from build123d import *
from build123d.topology import SkipClean

# Parameters (mm, degrees)
BOSS_EXTRUDE1_DEPTH      = 20
CUT_EXTRUDE1_DEPTH       = 60.487961127
BOSS_EXTRUDE2_DEPTH      = 4
CHAMFER1_SIZE            = 4
BOSS_EXTRUDE3_DEPTH      = 30
BOSS_EXTRUDE3_DEPTH_BACK = 80
CUT_EXTRUDE2_DEPTH       = 163.896367878
SHELL1_START             = -17.663350197
SHELL1_DEPTH             = 97.938189841
SHELL1_START_2           = -19.725064534
SHELL1_2_OUTLINE_W       = 18
SHELL1_2_OUTLINE_H       = 46
SHELL1_2_DEPTH           = 3.170813997
SHELL1_START_3           = 4.138253986
SHELL1_3_DEPTH           = 15.861746014
SHELL1_START_4           = -11.021607192
SHELL1_4_DEPTH           = 5.325277307
SHELL1_START_5           = -5.696329885
SHELL1_5_DEPTH           = 2


with BuildPart() as part:
    # Sketch1 → Boss-Extrude1 (new body)
    with BuildSketch(Plane(origin=(0, 0, 0), x_dir=(1, 0, 0), z_dir=(0, 1, 0))):
        with BuildLine():
            Line((25.274839644, -23.491941756), (25.274839644, 16.508058244))
            Line((25.274839644, 16.508058244), (-18.05582698, 16.508058244))
            ThreePointArc((-18.05582698, 16.508058244), (-21.573303396, -3.353843819), (-20.422301498, -23.491941756))
            ThreePointArc((-20.422301498, -23.491941756), (-19.386839701, -28.526912443), (-18.05582698, -33.491941756))
            Line((-18.05582698, -33.491941756), (25.274839644, -33.491941756))
            Line((25.274839644, -33.491941756), (25.274839644, -23.491941756))
        make_face()
    extrude(amount=BOSS_EXTRUDE1_DEPTH)

    # Sketch2 → Cut-Extrude1 (cut, through all)
    with BuildSketch(Plane.XY.offset(33.491941756)):
        Polygon((-18.05582698, 10), (-18.05582698, 0), (-8.05582698, 0), align=None)
        Polygon((-8.05582698, 0), (-18.05582698, 0), (-18.05582698, 10), (-26.022793605, 17.966966625), (-26.022793605, -4.913514026), (-8.05582698, -4.913514026), align=None)
    extrude(amount=-CUT_EXTRUDE1_DEPTH, mode=Mode.SUBTRACT)

    # Sketch3 → Boss-Extrude2 (add)
    with BuildSketch(Plane(origin=(0, 20, 0), x_dir=(1, 0, 0), z_dir=(0, 1, 0))):
        with BuildLine():
            Line((-20.591335302, 5.508058244), (-18.56429203, 5.508058244))
            ThreePointArc((-18.56429203, 5.508058244), (-19.725160356, -8.491941756), (-18.56429203, -22.491941756))
            Line((-18.56429203, -22.491941756), (-20.591335302, -22.491941756))
            ThreePointArc((-20.591335302, -22.491941756), (-21.725160356, -8.491941756), (-20.591335302, 5.508058244))
        make_face()
    extrude(amount=BOSS_EXTRUDE2_DEPTH)

    # Chamfer1
    chamfer1_edges = [part.edges().sort_by_distance(p)[0] for p in [
        (-19.577813666, 24, -5.508058244),
        (-19.577813666, 24, 22.491941756),
    ]]
    chamfer(chamfer1_edges, length=CHAMFER1_SIZE - 0.0001)  # a hair under: the kernel refuses the full size

    # Sketch4 → Boss-Extrude3 (add, two sides: drawn at the far end of the back side and taken through both)
    with BuildSketch(Plane.XY.offset(33.491941756).offset(-BOSS_EXTRUDE3_DEPTH_BACK)):
        Polygon((65.274839644, 110), (57.510268291, 81.022225211), (25.274839644, 20), (25.274839644, 0), (80.274839644, 0), (80.274839644, 110), align=None)
    extrude(amount=BOSS_EXTRUDE3_DEPTH + BOSS_EXTRUDE3_DEPTH_BACK)

    # Sketch5 → Cut-Extrude2 (cut, through all)
    with BuildSketch(Plane(origin=(80.274839644, 0, 0), x_dir=(0, 0, -1), z_dir=(1, 0, 0))):
        Polygon((-63.491941756, 0), (-33.491941756, 0), (-33.491941756, 30), (-63.491941756, 81.022225211), align=None)
    cut_extrude2 = extrude(amount=-CUT_EXTRUDE2_DEPTH, mode=Mode.SUBTRACT)

    # Mirror1: Cut-Extrude2 across plane
    add(cut_extrude2.mirror(Plane.XY.offset(8.491941756)), mode=Mode.SUBTRACT)

    # Shell1: read off the stored shape, not the designer's step
    # Shell1 outline → Shell1 (cut)
    with BuildSketch(Plane.YZ.offset(SHELL1_START)):
        Polygon((2, 31.491941756), (2, -14.508058244), (30.544412087, -14.508058244), (81.566637298, -44.508058244), (110, -44.508058244), (110, 61.491941756), (81.566637298, 61.491941756), (30.544412087, 31.491941756), align=None)
    extrude(amount=SHELL1_DEPTH, mode=Mode.SUBTRACT)

    # Shell1 2 outline → Shell1 2 (cut)
    with BuildSketch(Plane.YZ.offset(SHELL1_START_2)):
        with Locations((11, 8.491941756)):
            Rectangle(SHELL1_2_OUTLINE_W, SHELL1_2_OUTLINE_H)
    extrude(amount=SHELL1_2_DEPTH, mode=Mode.SUBTRACT)

    # Shell1 3 outline → Shell1 3 (add)
    with SkipClean():  # the faces are left unmerged after this step: merging them gives an invalid solid
        with BuildSketch(Plane(origin=(0, 0, 0), x_dir=(1, 0, 0), z_dir=(0, 1, 0)).offset(SHELL1_START_3)):
            with BuildLine():
                ThreePointArc((-19.725064534, -27.039617882), (-19.20680208, -29.272995907), (-18.62986821, -31.491941756))
                Line((-18.62986821, -31.491941756), (-16.554250537, -31.491941756))
                ThreePointArc((-16.554250537, -31.491941756), (-18.92870145, -20.100717198), (-19.725160356, -8.491941756))
                Line((-19.725160356, -8.491941756), (-19.725064534, -27.039617882))
            make_face()
            with BuildLine():
                ThreePointArc((-18.62986821, 14.508058244), (-19.20680208, 12.289112394), (-19.725064535, 10.055734369))
                Line((-19.725064535, 10.055734369), (-19.725160356, -8.491941756))
                ThreePointArc((-19.725160356, -8.491941756), (-18.92870145, 3.116833686), (-16.554250537, 14.508058244))
                Line((-16.554250537, 14.508058244), (-18.62986821, 14.508058244))
            make_face()
        extrude(amount=SHELL1_3_DEPTH)

    # Shell1 4 outline → Shell1 4 (cut)
    with SkipClean():  # the faces are left unmerged after this step: merging them gives an invalid solid
        with BuildSketch(Plane(origin=(0, 0, 0), x_dir=(0.7071067811865509, -0.707106781186544, 0), z_dir=(0.707106781186544, 0.707106781186551, 0)).offset(SHELL1_START_4)):
            with BuildLine():
                Line((-5.696329885, 16.508058244), (-19.838465509, 16.508058244))
                add(Edge.make_bspline(
                    [(-19.838465509, 16.508058244), (-30.445406654, -8.491941756), (-19.838465509, -33.491941756)],
                    knots=[2.850127051, 2.850127051, 2.850127051, 3.433058256, 3.433058256, 3.433058256], degree=2, weights=[1, 0.957823754, 1]))
                Line((-19.838465509, -33.491941756), (-5.696329885, -33.491941756))
                Line((-5.696329885, -33.491941756), (-5.696329885, 16.508058244))
            make_face()
        extrude(amount=SHELL1_4_DEPTH, mode=Mode.SUBTRACT)

    # Shell1 5 outline → Shell1 5 (add)
    with SkipClean():  # the faces are left unmerged after this step: merging them gives an invalid solid
        with BuildSketch(Plane(origin=(0, 0, 0), x_dir=(0.7071067811865509, -0.707106781186544, 0), z_dir=(0.707106781186544, 0.707106781186551, 0)).offset(SHELL1_START_5)):
            with BuildLine():
                Line((-6.52475701, -31.491941756), (-6.52475701, 14.508058244))
                Line((-6.52475701, 14.508058244), (-19.71491574, 14.508058244))
                add(Edge.make_bspline(
                    [(-19.71491574, 14.508058244), (-28.857373182, -8.491941756), (-19.71491574, -31.491941756)],
                    knots=[2.867588645, 2.867588645, 2.867588645, 3.415596662, 3.415596662, 3.415596662], degree=2, weights=[1, 0.962695179, 1]))
                Line((-19.71491574, -31.491941756), (-6.52475701, -31.491941756))
            make_face()
        extrude(amount=SHELL1_5_DEPTH)


solid = part.part
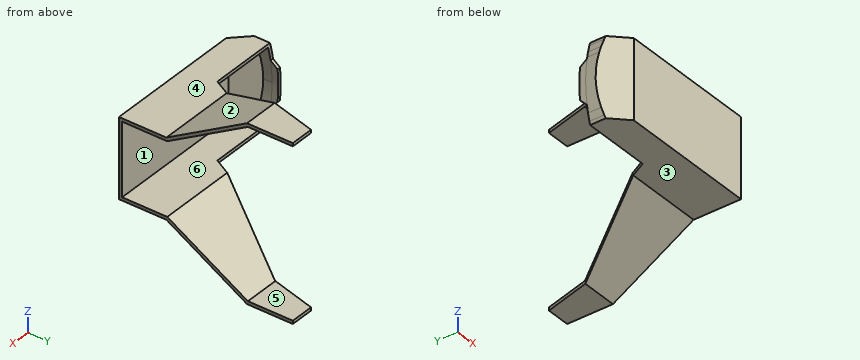
Input: part model. Units: mm. Frame: model coordinates. Face numbers are marked on the shaded views. A direction names the side the tool comes from. Coordinates: 2 decimals unless noted, no trailing zeros. Order: outer loops, then holes, each group sorted by start corner. A loop starts at its lowest first (then second) coordinate and runs counter-clockwise, first axis right, second up.
1. Access query for the marked faces 4, 5 and 6. Directions: +Z, -Z, +X, -X, +Y, -Y. A direction counts if a zero-diameter tool reaches every point of the face in a straight line with its end or side. Return the directions, or none.
Checked values:
face 4: +Z, +X, -X, -Y
face 5: +X, -X, +Y
face 6: +X, +Y
2. Cut plane B-B, the plane x = 23. Return loops of the section in (y, z), plus the area to 3 significant figures.
Checked values:
outline: (0, -16.51) - (20, -16.51) - (20, -14.51) - (2, -14.51) - (2, 31.49) - (20, 31.49) - (20, 33.49) - (0, 33.49) - close
area: 172 mm2
3. Contact query for flat-ended pins moving along their axis: P1, Ø5.5, axis at x = 9.5, z = -9, coming from the +Y side; P2, Ø15, axis at x = 9.5, y = 13, coming from the -Z side; P3, Ø1.5, axis at x = 56.5, y = 67.5, coming from the +Z side. Output: stop coordinate, or through.
Checked values:
P1: stops at y = 2
P2: stops at z = -16.51
P3: stops at z = 55.98
4. Cut plane C-C, the plane z = -8. Return loops of the section in (x, y).
Checked values:
outline: (-20.15, 12.09) - (-8.06, 0) - (80.27, 0) - (80.27, 2) - (-7.23, 2) - (-18.11, 12.88) - (-18.11, 20) - (-20.15, 20) - close
5. Cut plane D-D, the plane y = 21.5. Return loops of the section in (x, z), plus the area to 3 significant figures.
Checked values:
outline: (-20.82, -4.01) - (-18.8, -4.01) arc R85 cw to (-18.8, 20.99) - (-20.82, 20.99) arc R87 ccw to start; (26.07, -16.51) - (80.27, -16.51) - (80.27, -14.51) - (26.07, -14.51) - close; (26.07, 31.49) - (80.27, 31.49) - (80.27, 33.49) - (26.07, 33.49) - close
area: 267 mm2
6. Ray query, line 1 along Z through (x, y) = (75.5, 12); line 2 along Y through (x, z) = (23, 6.5); line 3 along Z through (x, y) = (73, 88). Return the intervals inside material, ascending.
Checked values:
line 1: z = -16.51 to -14.51, 31.49 to 33.49
line 2: y = 0 to 2
line 3: z = -46.51 to -44.51, 61.49 to 63.49
7. Cut plane A-A, the plane y = 76. Return loops of the section in (x, z) (3 decimals).
Checked values:
outline: (54.857, -43.555) - (80.275, -43.555) - (80.275, -41.235) - (54.857, -41.235) - close; (54.857, 58.219) - (80.275, 58.219) - (80.275, 60.539) - (54.857, 60.539) - close
8. Draft query along Z for the marked faces 1, 2 and 3. Return one class per face: +Z half, -Z half, draft (parallel to the pull), parting line (faces both ways), or undercut.
Checked values:
face 1: undercut
face 2: +Z half
face 3: -Z half
